from build123d import *

# Parameters (mm, degrees)
SKETCH1_W           = 640
SKETCH1_H           = 960
BOSS_EXTRUDE1_DEPTH = 42
SKETCH2_R           = 150
SKETCH2_R_2         = 90
BOSS_EXTRUDE2_DEPTH = 640
FILLET1_R           = 100
SKETCH3_W           = 280
SKETCH3_H           = 331.142467373
CUT_EXTRUDE1_DEPTH  = 1053


with BuildPart() as part:
    # Sketch1 → Boss-Extrude1 (new body)
    with BuildSketch(Plane.XY):
        with Locations((320, -480)):
            Rectangle(SKETCH1_W, SKETCH1_H)
    extrude(amount=BOSS_EXTRUDE1_DEPTH)

    # Sketch2 → Boss-Extrude2 (add)
    with BuildSketch(Plane.ZY):
        with Locations((162, -150)):
            Circle(SKETCH2_R)
        with Locations(Location((162, -150, 0), (0, 0, 270))):
            Circle(SKETCH2_R_2, mode=Mode.SUBTRACT)
    extrude(amount=-BOSS_EXTRUDE2_DEPTH)

    # Fillet1
    # the kernel refuses this fillet: 100 mm, written as the material it adds along each edge
    with BuildSketch(Plane(origin=(640, -240, 42), x_dir=(0, -0.48266089642206267, 0.8758073184582617), z_dir=(-1, 0, 0))) as fillet1_piece_1:
        with BuildLine():
            CenterArc((164.419726765, -91.161310821), FILLET1_R, 114.270768309, 94.588565736)
            Line((76.83899492, -139.427400463), (75.087380283, -140.392722256))
            Line((75.087380283, -140.392722256), (-1.751614637, -0.965321793))
            Line((-1.751614637, -0.965321793), (0.822098634, 1.823226216))
            ThreePointArc((0.822098634, 1.823226216), (61.657397537, -11.258033768), (122.49269644, 1.823226216))
            Line((122.49269644, 1.823226216), (123.314795074, 0))
        make_face()
    extrude(amount=640)
    with BuildSketch(Plane(origin=(640, -60, 42), x_dir=(0, 1, 0), z_dir=(-1, 0, 0))) as fillet1_piece_2:
        with BuildLine():
            CenterArc((148.795078393, -45.993847992), FILLET1_R, 152.616862204, 44.602125316)
            Line((53.277047036, -75.596308795), (51.366686409, -76.188358011))
            ThreePointArc((51.366686409, -76.188358011), (30.975334969, -34.741755066), (-1.2, -1.6))
            Line((-1.2, -1.6), (0, 2))
            ThreePointArc((0, 2), (30, 2), (58.224098432, 0.91987696))
            Line((58.224098432, 0.91987696), (60, 0))
        make_face()
    extrude(amount=640)

    # Sketch3 → Cut-Extrude1 (cut)
    with BuildSketch(Plane.XZ.offset(960)):
        with Locations((320, 207.571233687)):
            Rectangle(SKETCH3_W, SKETCH3_H)
    extrude(amount=-CUT_EXTRUDE1_DEPTH, mode=Mode.SUBTRACT)


solid = part.part
Can you work these out from the model? Positions are in its coordinate system, mm. A direction names the side the tool comes from. Round coordinates to 2 decimals unless told otherwise and drop trailing zeros. Order: outer loops, then holes, each group sorted by start corner. A loop starts at its lowest first (then second) coordinate and runs counter-clockwise, first axis right, second up. Notation, with made-up numbers: (71.25, -19.5) - (106.25, -19.5) arc R20 cw to (106.25, -1.5) - close; hole circle Ø7 at (6, -26.5). An arc over 180 degrees is marked (long way). Answer in a Markdown table with one row per item.
(1) Please list where these lines run through material, in increasing order: L1, parallel to X at y = -334.5, z = 43.5; L2, parallel to Z at x = 55, y = -150; L3, parallel to Z at x = 235, y = -919. Write a range as from..to.
From the geometry:
| item | result |
|---|---|
| L1 | x = 0..180, 460..640 |
| L2 | z = 0..72, 252..312 |
| L3 | z = 0..42 |
(2) Which directions (+Z, -Z, +X, -X, +Y, -Y) give clear straight access to the entire face, cutting with the end or side of a thin tool? Please do faces 5 (the face through (88.74, -130.49, 74.14)), 6 (the face through (316, -593, 42)), 7 (the face through (180, -202, 85)).
From the geometry:
| item | result |
|---|---|
| face 5 | +X, -X |
| face 6 | +Z, -Y |
| face 7 | +Z, +Y, -Y |
(3) For P1, Ø8, axis at x = 489.5, y = -125.5, coming from the -Z side; P2, Ø1.5, axis at x = 521.5, y = -852, coming from the +Z side; P3, Ø2, axis at x = 476, y = -208.5, coming from the +Z side; P4, Ø1, axis at x = 136, z = 121, coming from the -Y side, each with a flat end and sliding along its axis, tell me the tip position at first contact or that it passes through.
From the geometry:
| item | result |
|---|---|
| P1 | stops at z = 0 |
| P2 | stops at z = 42 |
| P3 | stops at z = 300.54 |
| P4 | stops at y = -301.54 |
(4) Suppose I cut it at D-D, the plane y = -847.5. Please give me the cut outline in (x, z).
From the geometry:
| item | result |
|---|---|
| outline | (0, 0) - (640, 0) - (640, 42) - (0, 42) - close |
(5) Suppose I cut it at B-B, the plane z = 162. Please give me the cut outline in (x, y), plus the area to 3 significant figures.
From the geometry:
| item | result |
|---|---|
| outline | (0, -300) - (180, -300) - (180, -240) - (0, -240) - close; (0, -60) - (180, -60) - (180, 0) - (0, 0) - close; (460, -300) - (640, -300) - (640, -240) - (460, -240) - close; (460, -60) - (640, -60) - (640, 0) - (460, 0) - close |
| area | 43,200 mm2 |
(6) Suppose I cut it at A-A, the plane y = -150. Please give me the cut outline in (x, z).
From the geometry:
| item | result |
|---|---|
| outline | (0, 0) - (640, 0) - (640, 72) - (460, 72) - (460, 42) - (180, 42) - (180, 72) - (0, 72) - close; (0, 252) - (180, 252) - (180, 312) - (0, 312) - close; (460, 252) - (640, 252) - (640, 312) - (460, 312) - close |
(7) If we mould it in two halves opening along Y, with no side actions, what happens to faces 1 (the face through (316, 0, 21)), 2 (the face through (91.26, -324.935, 75.03)), 3 (the face through (460, -202, 85)), 4 (the face through (548.74, -130.49, 74.14))? For each: released by +Y, released by -Y, zero draft, split by the parting line, or undercut.
From the geometry:
| item | result |
|---|---|
| face 1 | released by +Y |
| face 2 | released by -Y |
| face 3 | zero draft |
| face 4 | undercut |
(8) Suppose I cut it at C-C, the plane x = 114. Please give me the cut outline in (y, z).
From the geometry:
| item | result |
|---|---|
| outline | (-960, 0) - (0, 0) - (0, 42) arc R100 cw to (-6.72, 117.6) arc R150 ccw (long way) to (-299.52, 150) arc R100 cw to (-399.2, 42) - (-960, 42) - close; hole circle Ø180 at (-150, 162) |
